from build123d import *


with BuildPart() as part:
    # Sketch1 → Revolve1 (revolve)
    with BuildSketch(Plane.XY):
        Polygon((0, 38), (5, 38), (5, 15), (20, 15), (20, 0), (0, 0), align=None)
    revolve1 = revolve(axis=Axis((0, 0, 0), (0, 1, 0)))

    # Mirror1: Revolve1 across plane
    add(revolve1.mirror(Plane(origin=(20, 0, 0), x_dir=(0, 0, 1), z_dir=(0, -1, 0))))


solid = part.part
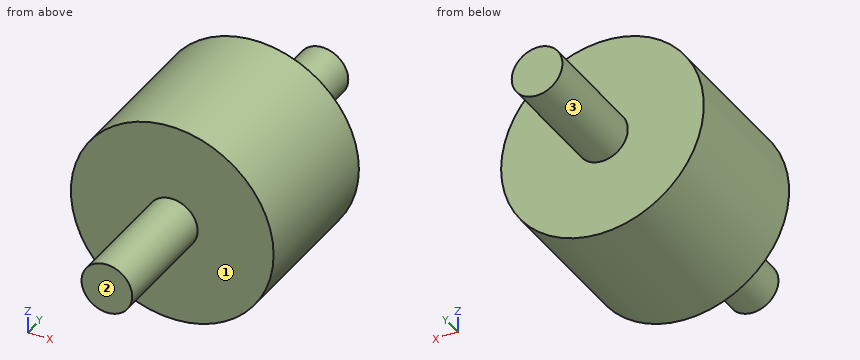
The model under review builds one solid part; all positions refer to its coordinate system, in mm. Face numbers are marked on the shaded views. A direction names the side the tool comes from. Round coordinates to 2 decimals unless told otherwise and drop trailing zeros. Order: outer loops, then holes, each group sorted by start corner. A loop starts at its lowest first (then second) coordinate and runs counter-clockwise, first axis right, second up. Notation, with made-up numbers: (32, 53) -> (54, 53) arc R16 ccw to (54, 84) -> close; hole circle Ø10 at (88.25, 48.25). An arc over 180 degrees is marked (long way). Write item = value, one per line. Start each with the question number.
Item 1: For line 1 along Y through (x, z) = (7, -9.5); line 2 along X through (y, z) = (-4, -3.5); line 3 along Z through (x, y) = (0, 12), list the stretches that pass through material, from the lowest coordinate up.
Item 2: Consider section B-B on x = 0. Write out the cut boundary in (y, z), plus the area to 3 significant figures.
Item 3: For the marked faces 1, 2 and 3, list the 3-axis set-ups (+Z, -Z, +X, -X, +Y, -Y) from which the entire face can be reached by the end or side of a thin tool; tool diameter is ignored.
Item 4: Consider section C-C on y = 7. Write out the cut boundary in (x, z).
Item 5: Consider section D-D on z = -12. Write out the cut boundary in (x, y), plus the area to 3 significant figures.
Item 6: Clearance check with flat-ended pins moving along their axes: pin 1 Ø12 at (x, z) = (-4.5, 3.5) entering from +Y; pin 2 Ø1 at (x, z) = (13, -10.5) entering from -Y; pin 3 Ø2 at (x, y) = (-0.5, -2) entering from -Z; pin 4 Ø8 at (x, y) = (1, -1.5) entering from +Z. State where each tip first meets the part, or that it passes through.
Item 7: Consider section A-A on z = 0. Write out the cut boundary in (x, y), plus the area to 3 significant figures.
Conclusion:
q1.line_1 = -15 to 15
q1.line_2 = -19.69 to 19.69
q1.line_3 = -20 to 20
q2.outline = (-38, -5) -> (-15, -5) -> (-15, -20) -> (15, -20) -> (15, -5) -> (38, -5) -> (38, 5) -> (15, 5) -> (15, 20) -> (-15, 20) -> (-15, 5) -> (-38, 5) -> close
q2.area = 1,660 mm2
q3.face_1 = -Y
q3.face_2 = +Z, -Z, +X, -X, -Y
q3.face_3 = +Y
q4.outline = circle Ø40 at (0, 0)
q5.outline = (-16, -15) -> (16, -15) -> (16, 15) -> (-16, 15) -> close
q5.area = 960 mm2
q6.pin_1 = 38
q6.pin_2 = -15
q6.pin_3 = -20
q6.pin_4 = 20
q7.outline = (-20, -15) -> (-5, -15) -> (-5, -38) -> (5, -38) -> (5, -15) -> (20, -15) -> (20, 15) -> (5, 15) -> (5, 38) -> (-5, 38) -> (-5, 15) -> (-20, 15) -> close
q7.area = 1,660 mm2
